Autodesk Inventor part; units mm, degrees
ref_plane "YZ Plane" through (0, 0, 0) normal (1, 0, 0) x (0, 1, 0)
ref_plane "XZ Plane" through (0, 0, 0) normal (0, 1, 0) x (-1, 0, 0)
ref_plane "XY Plane" through (0, 0, 0) normal (0, 0, 1) x (1, 0, 0)
sketch "Sketch2" plane through (0, 0, 0) normal (0, 0, 1) x (1, 0, 0)
  circle A0 centre (0, 0) radius 45
  dimension "d0" = 90
extrude "Extrusion1" add sketch "Sketch2" along normal blind 10
sketch "Sketch4" plane through (0, 0, 10) normal (0, 0, 1) x (1, 0, 0)
  circle A0 centre (0, 0) radius 11.5
  dimension "d14" = 23
extrude "Extrusion3" add sketch "Sketch4" along normal blind 23
sketch "Sketch5" plane through (0, 0, 33) normal (0, 0, 1) x (1, 0, 0)
  circle A0 centre (-8, 0) radius 2
  circle A1 centre (0, 0) radius 3.5
  circle A2 centre (0, 0) radius 11.5 construction
  circle A3 centre (-2.4721, -7.6085) radius 2
  circle A4 centre (6.4721, -4.7023) radius 2
  circle A5 centre (6.4721, 4.7023) radius 2
  circle A6 centre (-2.4721, 7.6085) radius 2
  dimension "d19" = 4
  dimension "d20" = 8
  dimension "d21" = 360
  dimension "d22" = 7
extrude "Extrusion4" cut sketch "Sketch5" against normal through all
sketch "Sketch8" plane through (0, 0, 33) normal (0, 0, 1) x (1, 0, 0)
  circle A0 centre (2.0086, 6.1819) radius 0.75
  circle A1 centre (-5.2586, 3.8206) radius 0.75
  circle A2 centre (-5.2586, -3.8206) radius 0.75
  circle A3 centre (2.0086, -6.1819) radius 0.75
  circle A4 centre (6.5, 0) radius 0.75
  circle A5 centre (-2.4721, 7.6085) radius 2 construction
  circle A6 centre (6.4721, 4.7023) radius 2 construction
  circle A7 centre (-2.4721, 7.6085) radius 2
  line L0 (6.4721, 4.7023) -> (-2.4721, 7.6085) construction
  line L1 (0, 0) -> (2.0086, 6.1819) construction
  point P0 (2, 6.1554)
  dimension "d44" = 1.5
  dimension "d45" = 6.5
  dimension "d48" = 360
extrude "Extrusion7" cut sketch "Sketch8" against normal through all contours A0 | A1 | A2 | A3 | A4
sketch "Sketch9" plane through (0, 0, 10) normal (0, 0, 1) x (1, 0, 0)
  circle A0 centre (0, 0) radius 22
  circle A1 centre (0, 0) radius 38
  dimension "d52" = 44
  dimension "d53" = 76
extrude "Extrusion8" cut sketch "Sketch9" against normal blind 7.35
sketch "Sketch10" plane through (0, 0, 0) normal (0, 0, -1) x (-1, 0, 0)
  circle A0 centre (0, 0) radius 22 construction
  circle A1 centre (0, 0) radius 38 construction
  circle A2 centre (0, 0) radius 22 construction
  circle A3 centre (0, 0) radius 38 construction
  circle A4 centre (15, 0) radius 1.25
  circle A5 centre (12.9904, 7.5) radius 1.25
  circle A6 centre (7.5, 12.9904) radius 1.25
  circle A7 centre (0, 15) radius 1.25
  circle A8 centre (-7.5, 12.9904) radius 1.25
  circle A9 centre (-12.9904, 7.5) radius 1.25
  circle A10 centre (-15, 0) radius 1.25
  circle A11 centre (-12.9904, -7.5) radius 1.25
  circle A12 centre (-7.5, -12.9904) radius 1.25
  circle A13 centre (0, -15) radius 1.25
  circle A14 centre (7.5, -12.9904) radius 1.25
  circle A15 centre (12.9904, -7.5) radius 1.25
  dimension "d56" = 2.5
  dimension "d59" = 360
  dimension "d66" = 15
extrude "Extrusion9" cut sketch "Sketch10" against normal through all
sketch "Sketch13" plane through (0, 0, 10) normal (0, 0, 1) x (1, 0, 0)
  circle A0 centre (0, 0) radius 45
  circle A1 centre (0, 0) radius 38
extrude "Extrusion10" add sketch "Sketch13" along normal blind 10
sketch "Sketch14" plane through (0, 0, 2.65) normal (0, 0, 1) x (1, 0, 0)
  circle A0 centre (0, 0) radius 22
  circle A1 centre (0, 0) radius 11.5
extrude "Extrusion11" cut sketch "Sketch14" along normal up to surface (7.35 mm away) from surface at 0
properties part number "SG02" material "ABS Plastic"
Model file for the job. Use its own axes, mm. A direction names the side the tool comes from. Round coordinates to 2 decimals unless told otherwise and drop trailing zeros. Loops run counter-clockwise (first coordinate to the right, second up) from the corner with the lowest first, then second, coordinate; pieces in that order, holes last. Notation, with made-up numbers: M 17.25,40 L 65.25,40 A5 cw 65.25,44 Z; hole C -11.5,52.5 d5. An arc over 180 degrees is marked long. Put each result on its own line as item: value. Start each with the question number.
Item 1: Drop flat-ended pins along their axis: P1, Ø2.5, axis at x = 2.01, y = 6.18, coming from the +Z side; P2, Ø4, axis at x = -12.99, y = -7.5, coming from the +Z side; P3, Ø2, axis at x = -21.5, z = 13.5, coming from the -Y side; P4, Ø10, axis at y = -33, z = 10.5, coming from the +X side. Give the stop position or say it passes through.
Item 2: Cut at D-D (x = 19.5). List the corners of the cut face in (y, z).
Item 3: Drill centre lines: line 1 along Y through (x, z) = (0, 1); line 2 along Y through (x, z) = (3, 16); line 3 along Y through (x, z) = (6.5, 14). Where is each one in solid material? Low to high.
Item 4: Cut at B-B (x = -7.5). List the corners of the cut face in (y, z), then the cut area to 3 significant figures.
Item 5: 3-axis set-ups, long thin cutter, end or side, ignore diameter. For faces 1 (the face through (-13.75, 0.05, 1.31)), 2 (the face through (17.535, 33.713, 11.204)): which of +Z, -Z, +X, -X, +Y, -Y reach the whole face in a straight line?
Item 6: Cut at A-A (z = 11). Give the number of separate pieces and of enclosed holes in the cut face, then the cut area to 3 significant figures.
Item 7: Cut at C-C (y = -30). List the corners of the cut face in (x, z).
Item 8: Mould opens along Y. For faces 3 (the face through (-0.6, -9.4, 0)), 4 (the face through (20.765, 39.923, 9.86)), 5 (the face through (-7.23, 11.77, 1.31)) say: released by +Y, released by -Y, zero draft, split by the parting line, or undercut.
Answer block:
1. P1: z = 33
1. P2: z = 2.65
1. P3: y = -40.06
1. P4: x = 35.23
2. outline: M -40.56,0 L 40.56,0 L 40.56,20 L 32.62,20 L 32.62,2.65 L -32.62,2.65 L -32.62,20 L -40.56,20 Z
3. line 1: -45 to -16.25, -13.75 to -3.5, 3.5 to 13.75, 16.25 to 45
3. line 2: -44.9 to -37.88, -11.1 to -1.8, 1.8 to 11.1, 37.88 to 44.9
3. line 3: -44.53 to -37.44, -9.49 to -6.7, -2.7 to -0.75, 0.75 to 2.7, 6.7 to 9.49, 37.44 to 44.53
4. outline: M -44.37,0 L -14.24,0 L -14.24,2.65 L -37.25,2.65 L -37.25,20 L -44.37,20 Z; M -11.74,0 L -1.94,0 L -1.94,33 L -8.72,33 L -8.72,2.65 L -11.74,2.65 Z; M 1.94,0 L 11.74,0 L 11.74,2.65 L 8.72,2.65 L 8.72,33 L 1.94,33 Z; M 14.24,0 L 44.37,0 L 44.37,20 L 37.25,20 L 37.25,2.65 L 14.24,2.65 Z
4. area: 870 mm2
5. face 1: +Z, -Z
5. face 2: +Z
6. separate pieces: 2
6. enclosed holes: 12
6. area: 2,130 mm2
7. outline: M -33.54,0 L 33.54,0 L 33.54,20 L 23.32,20 L 23.32,2.65 L -23.32,2.65 L -23.32,20 L -33.54,20 Z
8. face 3: zero draft
8. face 4: split by the parting line
8. face 5: undercut
